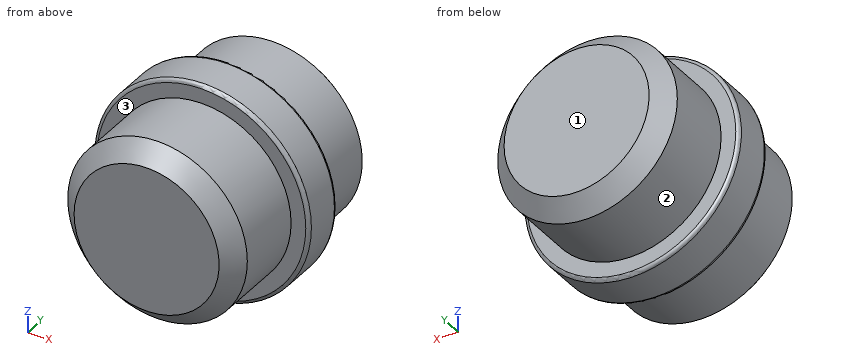
Autodesk Inventor part; units mm, degrees
ref_plane "YZ Plane" through (0, 0, 0) normal (1, 0, 0) x (0, 1, 0)
ref_plane "XZ Plane" through (0, 0, 0) normal (0, 1, 0) x (-1, 0, 0)
ref_plane "XY Plane" through (0, 0, 0) normal (0, 0, 1) x (1, 0, 0)
sketch "草图1" plane through (0, 0, 0) normal (0, 1, 0) x (-1, 0, 0)
  circle A0 centre (0, 0) radius 10.4
  dimension "d1" = 20.8
extrude "拉伸1" add sketch "草图1" along normal blind 10
sketch "草图2" plane through (0, 10, 0) normal (0, 1, 0) x (1, 0, 0)
  circle A0 centre (0, 0) radius 12.5
  dimension "d4" = 25
extrude "拉伸2" add sketch "草图2" along normal blind 5
sketch "草图3" plane through (0, 15, 0) normal (0, 1, 0) x (1, 0, 0)
  circle A0 centre (0, 0) radius 10.4
  dimension "d7" = 20.8
extrude "拉伸3" add sketch "草图3" along normal blind 10
chamfer "倒角1" distance 2 angle 45 2 edges at (10.4, 0, 0) (-10.4, 25, 0)
fillet "圆角1" radius 0.4 2 edges at (-12.5, 10, 0) (-12.5, 15, 0)
properties part number "GuardStopper"
Input: part model. Units: mm. Frame: model coordinates. Face numbers are marked on the shaded views. A direction names the side the tool comes from. Give positions to 0.01 mm unless a question says otherwise; leave off trailing zeros. Order: outer loops, then holes, each group sorted by start corner. A loop starts at its lowest first (then second) coordinate and runs counter-clockwise, first axis right, second up. Notation, with made-up numbers: (21.25, -26) - (53.25, -26) arc R13 ccw to (53.25, -2) - close; hole circle Ø10 at (-6.75, 41). An arc over 180 degrees is marked (long way). Answer as a JSON object with one key per item and string values. Group by question number.
Q1. Set-up query: the marked faces 1, 2 and 3. Return all of +Z, -Z, +X, -X, +Y, -Y with unobstructed straight access to the full face (end or side cutting, diameter ignored); none if empty.
Q2. First-contact query: pin 1 Ø3 at (x, y) = (-0.5, 18.5) entering from +Z; pin 2 Ø5 at (x, y) = (-9.5, 6) entering from +Z; pin 3 Ø2 at (y, z) = (22, -6.5) entering from -X. Flat tips, straight axial feed; report the tip coordinate or a pass-through.
Q3. Cut plane B-B, the plane x = 0. Output: boundary loops of the cut face in (y, z).
Q4. Line query: probe 1 along Y at (x, z) = (2.5, 10.5); probe 2 along Y at (x, z) = (3, -9); probe 3 along X at (y, z) = (8.25, -2). Output: solid intervals per line, ascending.
Q5. Cut plane D-D, the plane y = 11. Output: boundary loops of the cut face in (x, z).
Q6. Cut plane A-A, the plane z = 0. Output: boundary loops of the cut face in (x, y).
Q7. Cut plane C-C, the plane y = 5. Output: boundary loops of the cut face in (x, z).
Results:
{
 "1": {"face 1": "+Z, -Z, +X, -X, +Y", "face 2": "+Y", "face 3": "-Y"},
 "2": {"pin 1": "z = 10.4", "pin 2": "z = 7.69", "pin 3": "x = -8.83"},
 "3": {"outline": "(0, -8.4) - (2, -10.4) - (10, -10.4) - (10, -12.1) arc R0.4 ccw to (10.4, -12.5) - (14.6, -12.5) arc R0.4 ccw to (15, -12.1) - (15, -10.4) - (23, -10.4) - (25, -8.4) - (25, 8.4) - (23, 10.4) - (15, 10.4) - (15, 12.1) arc R0.4 ccw to (14.6, 12.5) - (10.4, 12.5) arc R0.4 ccw to (10, 12.1) - (10, 10.4) - (2, 10.4) - (0, 8.4) - close"},
 "4": {"probe 1": "10 to 15", "probe 2": "1.09 to 23.91", "probe 3": "-10.21 to 10.21"},
 "5": {"outline": "circle Ø25 at (0, 0)"},
 "6": {"outline": "(-12.5, 10.4) arc R0.4 ccw to (-12.1, 10) - (-10.4, 10) - (-10.4, 2) - (-8.4, 0) - (8.4, 0) - (10.4, 2) - (10.4, 10) - (12.1, 10) arc R0.4 ccw to (12.5, 10.4) - (12.5, 14.6) arc R0.4 ccw to (12.1, 15) - (10.4, 15) - (10.4, 23) - (8.4, 25) - (-8.4, 25) - (-10.4, 23) - (-10.4, 15) - (-12.1, 15) arc R0.4 ccw to (-12.5, 14.6) - close"},
 "7": {"outline": "circle Ø20.8 at (0, 0)"}
}
